Input: part model. Units: mm. Frame: model coordinates. Face numbers are marked on the shaded views. A direction names the side the tool comes from. Round coordinates to 2 decimals unless told otherwise and drop trailing zeros. Loops run counter-clockwise (first coordinate to the right, second up) from the corner with the lowest first, then second, coordinate; pieces in that order, holes last. Notation, with made-up numbers: (-20.75, -34) - (28.25, -34) arc R22 cw to (28.25, -2) - close; hole circle Ø11 at (41, 86.25). An arc over 180 degrees is marked (long way). One line per question, with ' | ' between items. Start each with the question number.
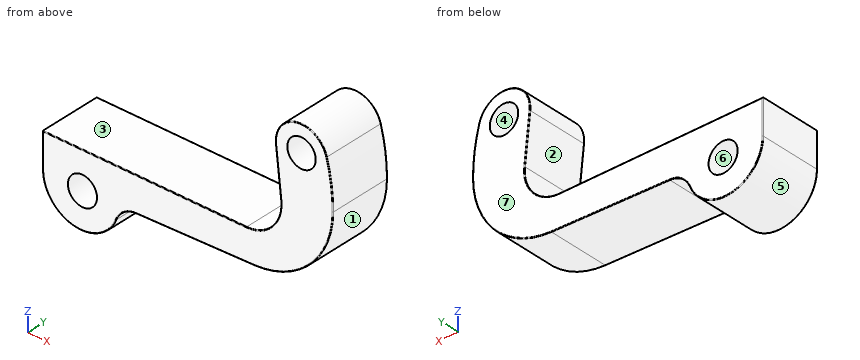
from build123d import *

# Parameters (mm, degrees)
SKETCH_1_R      = 4.1
SKETCH_1_R_2    = 4.2
EXTRUDE_1_DEPTH = 18
FILLET_1_R      = 0.2


with BuildPart() as part:
    # Эскиз1 → Бобышка-Вытянуть1 (new body)
    with BuildSketch(Plane(origin=(0, 0, 0), x_dir=(1, 0, 0), z_dir=(0, 1, 0))):
        with BuildLine():
            Line((0, 0), (58.849762768, 0))
            ThreePointArc((58.849762768, 0), (66.294383343, -3.323352301), (68.790784534, -11.084475102))
            Line((68.790784534, -11.084475102), (67.272727273, -25))
            ThreePointArc((67.272727273, -25), (73.338139081, -33.205921807), (82.0048561, -27.819421161))
            ThreePointArc((82.0048561, -27.819421161), (83.369847365, -21.141684374), (83.818322635, -14.340637419))
            ThreePointArc((83.818322635, -14.340637419), (77.194828854, 1.918929468), (61.12387315, 8.987774352))
            Line((61.12387315, 8.987774352), (26.92989503, 10))
            ThreePointArc((26.92989503, 10), (23.484932233, 11.148153988), (21.244623159, 14.005957604))
            ThreePointArc((21.244623159, 14.005957604), (8.961723124, 20.809506343), (0, 10))
            Line((0, 10), (0, 0))
        make_face()
        with Locations(Location((74.752421844, -25.81596668, 0), (0, 0, 270))):
            Circle(SKETCH_1_R, mode=Mode.SUBTRACT)
        with Locations(Location((11.5, 10.662869651, 0), (0, 0, 270))):
            Circle(SKETCH_1_R_2, mode=Mode.SUBTRACT)
    extrude(amount=EXTRUDE_1_DEPTH)

    # Скругление1
    fillet_1_edges = [part.edges().sort_by_distance(p)[0] for p in [
        (66.294383343, 18, 3.323352301),
        (44.02688409, 0, -9.493887176),
        (77.194828854, 0, -1.918929468),
        (83.369847365, 0, 21.141684374),
        (73.338139081, 0, 33.205921807),
        (68.031755904, 0, 18.042237551),
        (66.294383343, 0, 3.323352301),
        (29.424881384, 0, 0),
        (0, 0, -5),
        (68.031755904, 18, 18.042237551),
        (73.338139081, 18, 33.205921807),
        (83.369847365, 18, 21.141684374),
        (77.194828854, 18, -1.918929468),
        (44.02688409, 18, -9.493887176),
        (23.484932233, 18, -11.148153988),
        (8.961723124, 18, -20.809506343),
        (0, 18, -5),
        (29.424881384, 18, 0),
        (8.961723124, 0, -20.809506343),
        (23.484932233, 0, -11.148153988),
    ]]
    fillet(fillet_1_edges, radius=FILLET_1_R)


solid = part.part
(1) Section A-A, the plane y = 4.75. Output: boundary loops of the cut face in (x, z), plus the area to 3 significant figures.
(2) Pin query (flat end, axial travel): P1, Ø5, axis at x = 11.5, y = 15, coming from the +Z side; P2, Ø3, axis at x = 21.5, y = 3.5, coming from the -Z side; P3, Ø4, axis at y = 14, z = -13, coming from the -X side; P4, Ø5, axis at x = 74.75, z = 25.82, coming from the +Y side. Return the tip coordinate at first contact, or that it passes through.
(3) Line query: line 1 along X through (y, z) = (4.5, 25.5); line 2 along Z through (x, y) = (75, 8.25); line 3 along X through (y, z) = (5.25, 30). Output: solid intervals per line, ascending. Write a range as from..to.
(4) Pull-direction query (Z, two-part tool) for the marked faces 4, 5, 6 and 7; classes: released by +Z, released by -Z, zero draft, split by the parting line, or undercut.
(5) Reachability of the marked faces 1, 2 and 3 from +Z, -Z, +X, -X, +Y, -Y: full face, straight path, thin tool, end or side. Return the list, or none.
Derived:
1) outline: (0, -10) arc R11 ccw to (21.24, -14.01) arc R6.3 cw to (26.93, -10) - (61.12, -8.99) arc R23.39 ccw to (83.82, 14.34) arc R50.23 ccw to (82, 27.82) arc R7.52 ccw to (67.27, 25) - (68.79, 11.08) arc R10 cw to (58.85, 0) - (0, 0) - close; hole circle Ø8.4 at (11.5, -10.66); hole circle Ø8.2 at (74.75, 25.82) | area: 1,270 mm²
2) P1: stops at z = 0 | P2: stops at z = -16.32 | P3: stops at x = 0.05 | P4: passes through
3) line 1: x = 67.23..70.66, 78.84..82.59 | line 2: z = -3.91..21.72, 29.91..33.34 | line 3: x = 68.5..81.01
4) face 4: undercut | face 5: released by -Z | face 6: undercut | face 7: zero draft
5) face 1: -Z, +X, +Y, -Y | face 2: -X, +Y, -Y | face 3: +Z, -X, +Y, -Y
